```python
from build123d import *

# Parameters (mm, degrees)
SKETCH_1_W          = 48
SKETCH_1_H          = 35
EXTRUDE_1_DEPTH     = 5
SKETCH_2_W          = 41
SKETCH_2_H          = 30
CUT_EXTRUDE_1_DEPTH = 4
SKETCH_3_R          = 0.5
CUT_EXTRUDE_2_DEPTH = 6
SKETCH_4_R          = 1
CUT_EXTRUDE_5_DEPTH = 4
SKETCH_5_W          = 4
SKETCH_5_H          = 12
CUT_EXTRUDE_4_DEPTH = 6
CHAMFER_2_SIZE      = 4.9
CHAMFER_3_SIZE      = 1
CHAMFER_6_SIZE      = 2


with BuildPart() as part:
    # 草图1 → 凸台-拉伸1 (new body)
    with BuildSketch(Plane(origin=(0, 0, 0), x_dir=(1, 0, 0), z_dir=(0, 1, 0))):
        Rectangle(SKETCH_1_W, SKETCH_1_H)
    extrude(amount=EXTRUDE_1_DEPTH)

    # 草图2 → 切除-拉伸1 (cut)
    with BuildSketch(Plane(origin=(0, 5, 0), x_dir=(1, 0, 0), z_dir=(0, 1, 0))):
        with Locations((0, -1)):
            Rectangle(SKETCH_2_W, SKETCH_2_H)
    extrude(amount=-CUT_EXTRUDE_1_DEPTH, mode=Mode.SUBTRACT)

    # 草图3 → 切除-拉伸2 (cut, through all)
    with BuildSketch(Plane(origin=(0, 5, 0), x_dir=(1, 0, 0), z_dir=(0, 1, 0))):
        with Locations((-22.5, 10.5)):
            Circle(SKETCH_3_R)
        with Locations((-22.5, -13.5)):
            Circle(SKETCH_3_R)
        with Locations((22.5, -13.5)):
            Circle(SKETCH_3_R)
        with Locations((22.5, 10.5)):
            Circle(SKETCH_3_R)
    extrude(amount=-CUT_EXTRUDE_2_DEPTH, mode=Mode.SUBTRACT)

    # 草图4 → 切除-拉伸5 (cut)
    with BuildSketch(Plane.XZ):
        with Locations((-22.5, -10.5)):
            Circle(SKETCH_4_R)
        with Locations((-22.5, 13.5)):
            Circle(SKETCH_4_R)
        with Locations((22.5, 13.5)):
            Circle(SKETCH_4_R)
        with Locations((22.5, -10.5)):
            Circle(SKETCH_4_R)
    extrude(amount=-CUT_EXTRUDE_5_DEPTH, mode=Mode.SUBTRACT)

    # 草图5 → 切除-拉伸4 (cut, through all)
    with BuildSketch(Plane(origin=(0, 5, 0), x_dir=(1, 0, 0), z_dir=(0, 1, 0))):
        with Locations((-22, 0.5)):
            Rectangle(SKETCH_5_W, SKETCH_5_H)
        with Locations((22, 0.5)):
            Rectangle(SKETCH_5_W, SKETCH_5_H)
    extrude(amount=-CUT_EXTRUDE_4_DEPTH, mode=Mode.SUBTRACT)

    # 倒角2
    chamfer_2_edges = [part.edges().sort_by_distance(p)[0] for p in [
        (0, 0, -17.5),
    ]]
    chamfer(chamfer_2_edges, length=CHAMFER_2_SIZE)

    # 倒角3
    chamfer_3_edges = [part.edges().sort_by_distance(p)[0] for p in [
        (0, 0, 17.5),
    ]]
    chamfer(chamfer_3_edges, length=CHAMFER_3_SIZE)

    # 倒角6
    chamfer_6_edges = [part.edges().sort_by_distance(p)[0] for p in [
        (0, 1, -14),
    ]]
    chamfer(chamfer_6_edges, length=CHAMFER_6_SIZE)


solid = part.part
```
Here's how the part is built. I have some questions about the finished solid (model axes, mm). A direction names the side the tool comes from. Give positions to 0.01 mm unless a question says otherwise; leave off trailing zeros. Loops run counter-clockwise (first coordinate to the right, second up) from the corner with the lowest first, then second, coordinate; pieces in that order, holes last. Notation, with made-up numbers: (-31.5, -22.75) -> (20.5, -22.75) arc R34 cw to (20.5, 12.25) -> close; hole circle Ø3 at (8, 64.5). An arc over 180 degrees is marked (long way). Use one line per item in the form item = value. Start each with the question number.
1) For P1, Ø1.8, axis at x = 22.5, z = 13.5, coming from the -Y side; P2, Ø0.5, axis at y = 0.5, z = -1, coming from the -X side; P3, Ø2, axis at y = 1.5, z = 1, coming from the +X side, each with a flat end and sliding along its axis, tell me the tip position at first contact or that it passes through.
2) Thinking about a two-plate mould opening in X: for faces 1 (the face through (24, 2, -11)), 2 (the face through (0, 0, 2)), 3 (the face through (22.977, 4.507, 13.35)), 4 (the face through (-22.038, 4.507, -10.308)), which applies, +X half, -X half, draft (parallel to the pull), parting line (faces both ways), or undercut?
3) Imagine slicing it at A-A (x = -22.5). Please give me the cut outline in (y, z), then the cut area to 3 significant figures.
4) Which directions (+Z, -Z, +X, -X, +Y, -Y) give clear straight access to the entire face, cutting with the end or side of a thin tool? Please do faces 5 (the face through (-22, 3, -6.5)), 6 (the face through (22.283, 1.972, 12.524)), 7 (the face through (0, 3, 16)), 8 (the face through (0, 3, 17.5)), 9 (the face through (24, 2, 12)).
5) Imagine slicing it at C-C (z = -13.5). Please give me the cut outline in (x, y), then the cut area to 3 significant figures.
6) Please list where these lines run through material, in increasing order: line 1 along X through (y, z) = (4.85, 13.5); line 2 along Z through (x, y) = (-22.5, 2.9); line 3 along Z through (x, y) = (-22.5, 4.85).
7) Imagine slicing it at B-B (z = 13.5). Please give me the cut outline in (x, y).
8) Imagine slicing it at D-D (x = -17). Please give me the cut outline in (y, z).
Check values:
q1.P1 = 4
q1.P2 = -20
q1.P3 = 20
q2.face_1 = +X half
q2.face_2 = draft
q2.face_3 = undercut
q2.face_4 = undercut
q3.outline = (0, -12.6) -> (4.9, -17.5) -> (5, -17.5) -> (5, -11) -> (4, -11) -> (4, -11.5) -> (0, -11.5) -> close; (0, -9.5) -> (4, -9.5) -> (4, -10) -> (5, -10) -> (5, -6.5) -> (0, -6.5) -> close; (0, 5.5) -> (5, 5.5) -> (5, 13) -> (4, 13) -> (4, 12.5) -> (0, 12.5) -> close; (0, 14.5) -> (4, 14.5) -> (4, 14) -> (5, 14) -> (5, 17.5) -> (1, 17.5) -> (0, 16.5) -> close
q3.area = 84.5 mm^2
q4.face_5 = -X, +Y, -Y
q4.face_6 = -Y
q4.face_7 = +Y
q4.face_8 = +Z, +X, -X, +Y, -Y
q4.face_9 = +Z, -Z, +X, +Y, -Y
q5.outline = (-24, 0.9) -> (24, 0.9) -> (24, 5) -> (20.5, 5) -> (20.5, 2.5) -> (-20.5, 2.5) -> (-20.5, 5) -> (-24, 5) -> close
q5.area = 94.3 mm^2
q6.line_1 = -24 to -23, -22 to -20.5, 20.5 to 22, 23 to 24
q6.line_2 = -15.5 to -11.5, -9.5 to -6.5, 5.5 to 12.5, 14.5 to 17.5
q6.line_3 = -17.45 to -11, -10 to -6.5, 5.5 to 13, 14 to 17.5
q7.outline = (-24, 0) -> (-23.5, 0) -> (-23.5, 4) -> (-23, 4) -> (-23, 5) -> (-24, 5) -> close; (-22, 4) -> (-21.5, 4) -> (-21.5, 0) -> (21.5, 0) -> (21.5, 4) -> (22, 4) -> (22, 5) -> (20.5, 5) -> (20.5, 1) -> (-20.5, 1) -> (-20.5, 5) -> (-22, 5) -> close; (23, 4) -> (23.5, 4) -> (23.5, 0) -> (24, 0) -> (24, 5) -> (23, 5) -> close
q8.outline = (0, -12.6) -> (4.9, -17.5) -> (5, -17.5) -> (5, -14) -> (3, -14) -> (1, -12) -> (1, 16) -> (5, 16) -> (5, 17.5) -> (1, 17.5) -> (0, 16.5) -> close
